Study the drawing (mm; zero at the part's minimum x, y, z) and answer. Coordinates: 2 decimals unless noted, no trailing zeros. Write each loop counter-clockwise with the first axis right and the second up, starting at its lowest first coordinate (ties: lowest second). Pieces come first, ordered by that corner, then holes. Notation, with made-up numbers: (41, 69) -> (58, 69) arc R16 ccw to (58, 84) -> close; hole circle Ø1 at (6, -40). An arc over 180 degrees is marked (long way). Write item = value, one per line. Start each with the question number.
1) Find the intervals of material crossed by line 1 along Y through (x, z) = (8, 5.5); line 2 along X through (y, z) = (35, 7.25); line 3 along X through (y, z) = (9.5, 17), in increasing order. Write a range as from..to.
2) Section A-A (y = 32) is taken. Determine the outline of the cut face in (x, z).
3) Section B-B (x = 52) is taken. Determine the outline of the cut face in (y, z), plus the area to 3 significant figures.
4) Section C-C (z = 7.5) is taken. Determine the outline of the cut face in (x, y), plus the area to 3 significant figures.
5) For a pull along Y with two mould halves and no side action, classify the marked faces 1, 2, 3 and 4 as released by +Y, released by -Y, zero draft, split by the parting line, or undercut.
6) A flat-ended cylindrical pin translates along its axis: pin 1 Ø4 at (x, y) = (8, 8) entering from -Z. Find the tip coordinate at first contact, or state that the pin passes through.
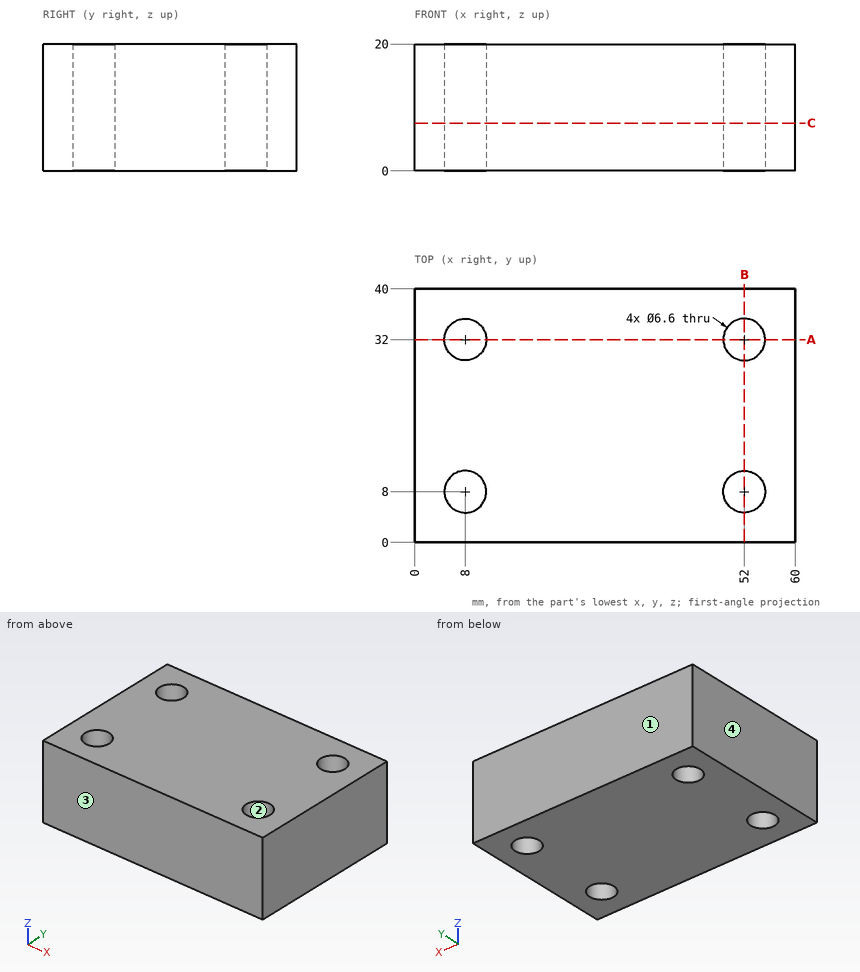
Answer key:
q1.line_1 = 0..4.7, 11.3..28.7, 35.3..40
q1.line_2 = 0..6.63, 9.37..50.63, 53.37..60
q1.line_3 = 0..5.06, 10.94..49.06, 54.94..60
q2.outline = (0, 0) -> (4.7, 0) -> (4.7, 20) -> (0, 20) -> close; (11.3, 0) -> (48.7, 0) -> (48.7, 20) -> (11.3, 20) -> close; (55.3, 0) -> (60, 0) -> (60, 20) -> (55.3, 20) -> close
q3.outline = (0, 0) -> (4.7, 0) -> (4.7, 20) -> (0, 20) -> close; (11.3, 0) -> (28.7, 0) -> (28.7, 20) -> (11.3, 20) -> close; (35.3, 0) -> (40, 0) -> (40, 20) -> (35.3, 20) -> close
q3.area = 536 mm^2
q4.outline = (0, 0) -> (60, 0) -> (60, 40) -> (0, 40) -> close; hole circle Ø6.6 at (8, 8); hole circle Ø6.6 at (8, 32); hole circle Ø6.6 at (52, 8); hole circle Ø6.6 at (52, 32)
q4.area = 2,260 mm^2
q5.face_1 = released by +Y
q5.face_2 = undercut
q5.face_3 = released by -Y
q5.face_4 = zero draft
q6.pin_1 = through
